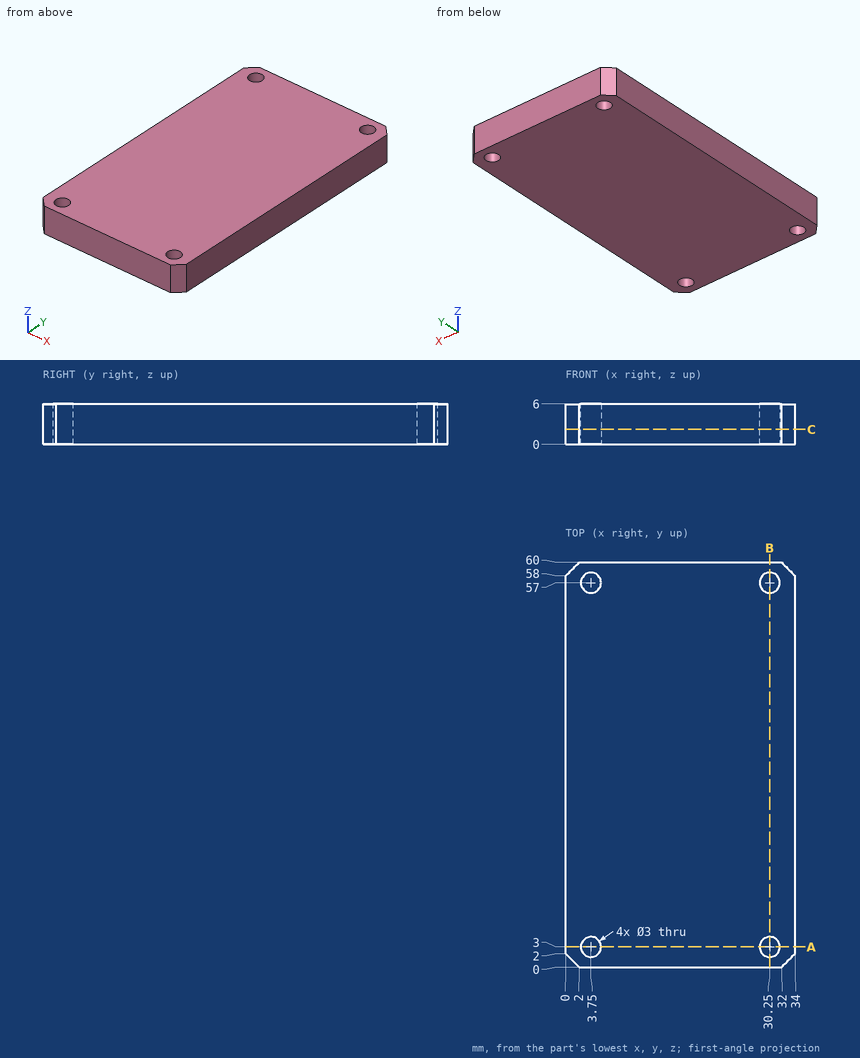
Source: three-view drawing plus pictorial views. Frame: mm from the lowest corner of the part. Give positions to 0.01 mm unless a question says otherwise; leave off trailing zeros. Order: outer loops, then holes, each group sorted by start corner. A loop starts at its lowest first (then second) coordinate and runs counter-clockwise, first axis right, second up. Notation, with made-up numbers: (10, -8) - (68, -8) arc R33 ccw to (68, 28) - close; hole circle Ø2 at (17.5, -11). An arc over 180 degrees is marked (long way). Put each result on its own line as item: value.
Item 1: Section query A-A, the plane y = 3. Return loops of the section in (x, z), then the cut area to 3 significant figures.
Found:
outline: (0, 0) - (2.25, 0) - (2.25, 6) - (0, 6) - close; (5.25, 0) - (28.75, 0) - (28.75, 6) - (5.25, 6) - close; (31.75, 0) - (34, 0) - (34, 6) - (31.75, 6) - close
area: 168 mm^2
Item 2: Section query B-B, the plane x = 30.25. Return loops of the section in (y, z), then the cut area to 3 significant figures.
Found:
outline: (0, 0) - (1.5, 0) - (1.5, 6) - (0, 6) - close; (4.5, 0) - (55.5, 0) - (55.5, 6) - (4.5, 6) - close; (58.5, 0) - (60, 0) - (60, 6) - (58.5, 6) - close
area: 324 mm^2
Item 3: Ray query, L1, parallel to Y at x = 30.25, z = 4.15; L2, parallel to Y at x = 3, z = 4. Return the intervals inside material, ascending. Write a range as from..to.
Found:
L1: y = 0..1.5, 4.5..55.5, 58.5..60
L2: y = 0..1.7, 4.3..55.7, 58.3..60
Item 4: Section query C-C, the plane z = 2.25. Return loops of the section in (x, y).
Found:
outline: (0, 2) - (2, 0) - (32, 0) - (34, 2) - (34, 58) - (32, 60) - (2, 60) - (0, 58) - close; hole circle Ø3 at (3.75, 3); hole circle Ø3 at (3.75, 57); hole circle Ø3 at (30.25, 3); hole circle Ø3 at (30.25, 57)
Item 5: Contact query for a flat-ended pin moving along its axis: pin 1 (3.5 mm diameter, centred on x = 3.75, y = 57, fed in from -Z). Output: stop coordinate, or through.
Found:
pin 1: stops at z = 0
